Can you work these out from the model? Positions are in its coordinate system, mm. Face numbers are marked on the shaded views. Give positions to 0.01 mm unless a question says otherwise; leave off trailing zeros. Write each loop counter-clockwise with the first axis right and the second up, starting at its lowest first coordinate (ties: lowest second). Pieces come first, ordered by that corner, then holes. Notation, with made-up numbers: (-5, 85) - (48, 85) arc R31 cw to (48, 120) - close; hole circle Ø10 at (8.5, 48.5). An arc over 180 degrees is marked (long way). Return JSON: item names as keys, results as strings. Group by question number.
from build123d import *

# Parameters (mm, degrees)
F1_DEPTH = 12.7508
F2_R     = 2.119579
F3_DEPTH = 12.7
F5_DEPTH = 12.7


with BuildPart() as f1:
    # F0 (on Top) → F1 (new body)
    with BuildSketch(Plane.XY):
        with BuildLine():
            Line((5.493004, 5.870853), (-5.493004, 5.870853))
            ThreePointArc((-5.493004, 5.870853), (-6.907215, 5.285067), (-7.493, 3.870857))
            Line((-7.493, 3.870857), (-7.493, -3.870857))
            ThreePointArc((-7.493, -3.870857), (-6.907215, -5.285067), (-5.493004, -5.870853))
            Line((-5.493004, -5.870853), (5.493004, -5.870853))
            ThreePointArc((5.493004, -5.870853), (6.907215, -5.285067), (7.493, -3.870857))
            Line((7.493, -3.870857), (7.493, 3.870857))
            ThreePointArc((7.493, 3.870857), (6.907215, 5.285067), (5.493004, 5.870853))
        make_face()
    extrude(amount=F1_DEPTH)

    # F2 (on face) → F3 (join)
    with BuildSketch(Plane.XY.offset(12.7508)):
        Circle(F2_R)
    extrude(amount=F3_DEPTH)

    # F4 (on face) → F5 (cut)
    with BuildSketch(Plane.XY.offset(25.4508)):
        with BuildLine():
            Line((2.119579, 0), (0, 0))
            Line((0, 0), (-2.119579, 0))
            ThreePointArc((-2.119579, 0), (0, -2.119579), (2.119579, 0))
        make_face()
    extrude(amount=-F5_DEPTH, mode=Mode.SUBTRACT)


solid = f1.part
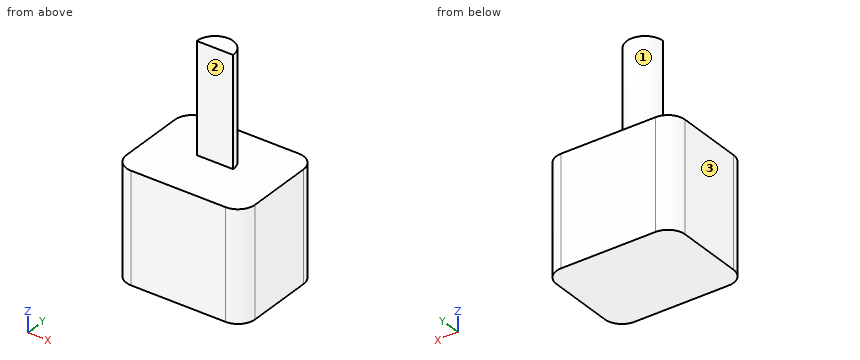
1) We'd pull the mould along X, two halves only. Please class the marked faces 1, 2 and 3: pulls with the +X half, pulls with the -X half, needs draft (parallel to the pull), parting line crosses it, or undercut.
2) Imagine slicing it at A-A, the plane z = 4. Write out the boundary of the cut face in (x, y), and give its area (3 significant figures).
3) Will these pins go through, and if not, where does the flat tip stop? pin 1 Ø1.5 at (x, y) = (-3.5, 4) entering from +Z; pin 2 Ø4.5 at (x, z) = (0, 17.5) entering from -Y; pin 3 Ø4 at (y, z) = (1, 22.5) entering from -X.
4) Imagine slicing it at B-B, the plane x = 0. Write out the boundary of the cut face in (y, z), and give its area (3 significant figures).
5) I need wall thicknesses on line 1 along Z through (x, y) = (3.75, -5.5); line 2 along Y through (x, z) = (0, 17.75); line 3 along X through (y, z) = (-4, 7). Which ranges of each line are inside material? Lowest first, please.
6) Imagine slicing it at C-C, the plane y = -1.5. Write out the boundary of the cut face in (x, z).
7) Imagine slicing it at D-D, the plane x = -3.25. Write out the boundary of the cut face in (y, z), and give its area (3 significant figures).
Resolved:
{
 "1": {"face 1": "parting line crosses it", "face 2": "needs draft", "face 3": "pulls with the -X half"},
 "2": {"outline": "(-7.49, -3.87) arc R2 ccw to (-5.49, -5.87) - (5.49, -5.87) arc R2 ccw to (7.49, -3.87) - (7.49, 3.87) arc R2 ccw to (5.49, 5.87) - (-5.49, 5.87) arc R2 ccw to (-7.49, 3.87) - close", "area": "173 mm^2"},
 "3": {"pin 1": "z = 12.75", "pin 2": "y = 0", "pin 3": "x = -2.12"},
 "4": {"outline": "(-5.87, 0) - (5.87, 0) - (5.87, 12.75) - (2.12, 12.75) - (2.12, 25.45) - (0, 25.45) - (0, 12.75) - (-5.87, 12.75) - close", "area": "177 mm^2"},
 "5": {"line 1": "0 to 12.75", "line 2": "0 to 2.12", "line 3": "-7.49 to 7.49"},
 "6": {"outline": "(-7.49, 0) - (7.49, 0) - (7.49, 12.75) - (-7.49, 12.75) - close"},
 "7": {"outline": "(-5.87, 0) - (5.87, 0) - (5.87, 12.75) - (-5.87, 12.75) - close", "area": "150 mm^2"}
}
